```python
from build123d import *

# Parameters (mm, degrees)
CYLINDER022_R          = 1.6
CYLINDER022_DEPTH      = 10
CYLINDER021_R          = 1.6
CYLINDER021_DEPTH      = 10
CYLINDER020_R          = 50
CYLINDER020_DEPTH      = 7.5
CYLINDER020_ROLL_ANGLE = 90
CYLINDER019_R          = 51
CYLINDER019_DEPTH      = 7.5
CYLINDER019_ROLL_ANGLE = 90
BOX022_W               = 317
BOX022_H               = 10
BOX022_DEPTH           = 300
CYLINDER018_R          = 50
CYLINDER018_DEPTH      = 7.5
CYLINDER018_ROLL_ANGLE = 90
CYLINDER017_R          = 4.75
CYLINDER017_DEPTH      = 1
CYLINDER016_R          = 4.75
CYLINDER016_DEPTH      = 1
BOX021_W               = 12
BOX021_H               = 7.5
BOX021_DEPTH           = 1


with BuildPart() as cylinder022:
    # Cylinder022 → Cylinder022 (new body)
    with BuildSketch(Plane(origin=(0, -18, -9.2), x_dir=(1, 0, 0), z_dir=(0, 0, 1))):
        Circle(CYLINDER022_R)
    extrude(amount=CYLINDER022_DEPTH)


with BuildPart() as fusion015:
    # Cylinder021 → Cylinder021 (new body)
    with BuildSketch(Plane(origin=(12, -18, -9.2), x_dir=(1, 0, 0), z_dir=(0, 0, 1))):
        Circle(CYLINDER021_R)
    extrude(amount=CYLINDER021_DEPTH)

    # Fusion015: union Cylinder022
    add(cylinder022.part)


with BuildPart() as fusion015_1:
    # Fusion015 placement: moved
    add(fusion015.part.moved(Location((0, 0, 5))))


with BuildPart() as cylinder020:
    # Cylinder020 → Cylinder020 (new body)
    with BuildSketch(Plane.XY):
        Circle(CYLINDER020_R)
    extrude(amount=CYLINDER020_DEPTH)


with BuildPart() as cylinder020_1:
    # Cylinder020 roll: moved
    add(cylinder020.part.rotate(Axis((0, 0, 0), (1, 0, 0)), CYLINDER020_ROLL_ANGLE))


with BuildPart() as cylinder020_2:
    # Cylinder020 placement: moved
    add(cylinder020_1.part.moved(Location((6, -14.25, 49.2))))


with BuildPart() as cut019:
    # Cylinder019 → Cylinder019 (new body)
    with BuildSketch(Plane.XY):
        Circle(CYLINDER019_R)
    extrude(amount=CYLINDER019_DEPTH)


with BuildPart() as cut019_1:
    # Cylinder019 roll: moved
    add(cut019.part.rotate(Axis((0, 0, 0), (1, 0, 0)), CYLINDER019_ROLL_ANGLE))


with BuildPart() as cut019_2:
    # Cylinder019 placement: moved
    add(cut019_1.part.moved(Location((6, -14.25, 49.2))))

    # Cut019: cut Cylinder020
    add(cylinder020_2.part, mode=Mode.SUBTRACT)


with BuildPart() as box022:
    # Box022 → Box022 (new body)
    with BuildSketch(Plane(origin=(-150, -22, 0), x_dir=(1, 0, 0), z_dir=(0, 0, 1))):
        with Locations((158.5, 5)):
            Rectangle(BOX022_W, BOX022_H)
    extrude(amount=BOX022_DEPTH)


with BuildPart() as cut018:
    # Cylinder018 → Cylinder018 (new body)
    with BuildSketch(Plane.XY):
        Circle(CYLINDER018_R)
    extrude(amount=CYLINDER018_DEPTH)


with BuildPart() as cut018_1:
    # Cylinder018 roll: moved
    add(cut018.part.rotate(Axis((0, 0, 0), (1, 0, 0)), CYLINDER018_ROLL_ANGLE))


with BuildPart() as cut018_2:
    # Cylinder018 placement: moved
    add(cut018_1.part.moved(Location((6, -14.25, 49.2))))

    # Cut018: cut Box022
    add(box022.part, mode=Mode.SUBTRACT)


with BuildPart() as cylinder017:
    # Cylinder017 → Cylinder017 (new body)
    with BuildSketch(Plane(origin=(0, -18, 0), x_dir=(1, 0, 0), z_dir=(0, 0, 1))):
        Circle(CYLINDER017_R)
    extrude(amount=CYLINDER017_DEPTH)


with BuildPart() as cylinder016:
    # Cylinder016 → Cylinder016 (new body)
    with BuildSketch(Plane(origin=(12, -18, 0), x_dir=(1, 0, 0), z_dir=(0, 0, 1))):
        Circle(CYLINDER016_R)
    extrude(amount=CYLINDER016_DEPTH)


with BuildPart() as obj1:
    # Box021 → Box021 (new body)
    with BuildSketch(Plane(origin=(0, -21.75, 0), x_dir=(1, 0, 0), z_dir=(0, 0, 1))):
        with Locations((6, 3.75)):
            Rectangle(BOX021_W, BOX021_H)
    extrude(amount=BOX021_DEPTH)

    # Fusion014: union Cut018, Cylinder017, Cylinder016
    add(cut018_2.part)
    add(cylinder017.part)
    add(cylinder016.part)

    # Cut020: cut Cut019
    add(cut019_2.part, mode=Mode.SUBTRACT)

    # Cut021: cut Fusion015
    add(fusion015_1.part, mode=Mode.SUBTRACT)


with BuildPart() as obj1_1:
    # Cut021 placement: moved
    add(obj1.part.moved(Location((92, 63, -38))))


solid = obj1_1.part
```
Can you work these out from the model? Positions are in its coordinate system, mm. A direction names the side the tool comes from. Give positions to 0.01 mm unless a question says otherwise; leave off trailing zeros. Order: outer loops, then holes, each group sorted by start corner. A loop starts at its lowest first (then second) coordinate and runs counter-clockwise, first axis right, second up. Notation, with made-up numbers: (68, 23) - (84, 23) arc R19 ccw to (84, 40) - close; hole circle Ø3 at (-1, -8.75). An arc over 180 degrees is marked (long way). Use a Markdown table: item, result. Add a question column.
Q1. I'm going to push flat-ended pins straight in: pin 1 (1.1 mm diameter, centred on x = 92, y = 49, fed in from -Z); pin 2 (4 mm diameter, centred on x = 90, y = 44.5, fed in from -Z); pin 3 (0.9 mm diameter, centred on x = 98, z = -38, fed in from -Y). Where does each tip first touch, or does it pass through?
Q2. On a 3-axis mill with a long thin cutter (end or side, diameter ignored), from which of +Z, -Z, +X, -X, +Y, -Y can I reach the whole of each face in a straight line? I mean faces 4 (the flat face through (92, 41, -38)), 5 (the flat face through (98, 41.25, -38)), 6 (the flat face through (92, 49, -38)). Say none if no direction works.
Q3. Please list where these lines run through material, in increasing order: line 1 along X through (y, z) = (45, -37.5); line 2 along Y through (x, z) = (92, -37.55); line 3 along X through (y, z) = (44, -37.55).
Q4. If we section it at B-B on y = 45: Write out the boundary of the cut face in (x, z), plus the area to 3 significant figures.
Q5. If we section it at A-A on z = -37.2: Write out the boundary of the cut face in (x, y), plus the area to 3 significant figures.
Q6. If we section it at C-C on x = 92: Write out the boundary of the cut face in (y, z).
Q7. If we mould it in two halves opening along X, with no side actions, what happens to faces 1 (the cylindrical face through (97.8, 45.1, -38.8)), 2 (the flat face through (104, 49, -38)), 3 (the cylindrical face through (102.4, 45.07, -37.64))? For each: released by +X, released by -X, zero draft, split by the parting line, or undercut.
Q8. If we section it at D-D on x = 97: Write out the boundary of the cut face in (y, z).
Answers follow:
| question | item | result |
|---|---|---|
| 1 | pin 1 | stops at z = -38.5 |
| 1 | pin 2 | stops at z = -38.4 |
| 1 | pin 3 | stops at y = 41.25 |
| 2 | face 4 | -Z, +X, -X, -Y |
| 2 | face 5 | -Z, -Y |
| 2 | face 6 | -Z, +X, -X, +Y |
| 3 | line 1 | x = 87.25 to 90.4, 93.6 to 102.4, 105.6 to 108.75 |
| 3 | line 2 | y = 40.25 to 43.4, 46.6 to 49.75 |
| 3 | line 3 | x = 87.36 to 90.75, 93.25 to 102.75, 105.25 to 108.64 |
| 4 | outline | (87.25, -37.63) arc R50 ccw to (90.4, -38.22) - (90.4, -37) - (87.25, -37) - close; (93.6, -38.61) arc R50 ccw to (102.4, -38.61) - (102.4, -37) - (93.6, -37) - close; (105.6, -38.22) arc R50 ccw to (108.75, -37.63) - (108.75, -37) - (105.6, -37) - close |
| 4 | area | 21.2 mm^2 |
| 5 | outline | (94.92, 41.25) - (101.08, 41.25) arc R4.75 ccw (long way) to (101.08, 48.75) - (94.92, 48.75) arc R4.75 ccw (long way) to start; hole circle Ø3.2 at (92, 45); hole circle Ø3.2 at (104, 45) |
| 5 | area | 153 mm^2 |
| 6 | outline | (40.25, -38) - (41.25, -38) - (41.25, -38.44) - (43.4, -38.44) - (43.4, -37) - (40.25, -37) - close; (46.6, -38.44) - (48.75, -38.44) - (48.75, -38) - (49.75, -38) - (49.75, -37) - (46.6, -37) - close |
| 7 | face 1 | split by the parting line |
| 7 | face 2 | zero draft |
| 7 | face 3 | undercut |
| 8 | outline | (41.25, -38.79) - (48.75, -38.79) - (48.75, -37) - (41.25, -37) - close |
